Part model, mm, in its own coordinate system. Give positions to 0.01 mm unless a question says otherwise; leave off trailing zeros. Order: outer loops, then holes, each group sorted by start corner. A loop starts at its lowest first (then second) coordinate and runs counter-clockwise, first axis right, second up.
1. Slice it at C-C on x = 50. List the corners of the cut face in (y, z), and give its area (3 significant figures).
2. Slice it at B-B on y = -62. List the corners of the cut face in (x, z).
3. Probe line 1 (Y direction, x = 0, z = 8.5); line 2 (Z direction, x = 46.5, y = 59); line 3 (X direction, y = 2, z = 3.5). List the from-to ranges inside material, lowest first.
4. Drop flat-ended pins along their axis: pin 1 Ø3 at (x, y) = (-45, -10) entering from +Z; pin 2 Ø3.5 at (x, z) = (-0.5, 4) entering from +Y. Give the stop position or say it passes through.
5. Slice it at A-A on z = 4.75. List the corners of the cut face in (x, y), and give its area (3 significant figures).
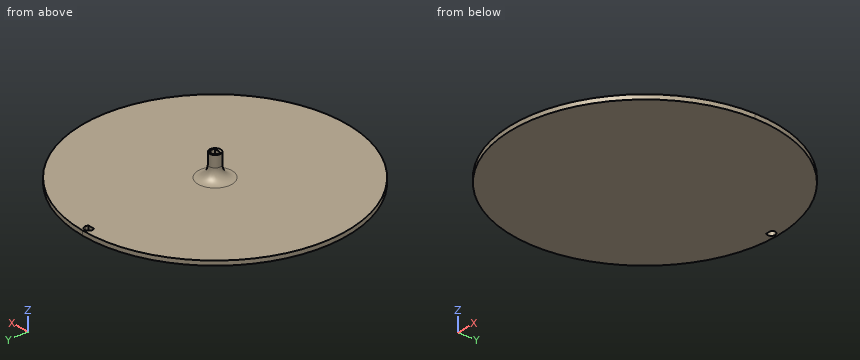
from build123d import *

# Parameters (mm, degrees)
F0_R     = 3.7
F1_DEPTH = 15
F3_DEPTH = 3


with BuildPart() as f1:
    # F0 (on Top) → F1 (new body)
    with BuildSketch(Plane.XY):
        Circle(F0_R)
        with BuildLine():
            ThreePointArc((-2.0976176963, -1.7), (-0.9017849577, 2.5449526302), (2.7, 0))
            ThreePointArc((2.7, 0), (2.5449526302, -0.9017849577), (2.0976176963, -1.7))
            ThreePointArc((2.0976176963, -1.7), (0, -2.7), (-2.0976176963, -1.7))
        make_face(mode=Mode.SUBTRACT)
        with BuildLine():
            Line((0, -1.7), (-2.0976176963, -1.7))
            ThreePointArc((-2.0976176963, -1.7), (0, -2.7), (2.0976176963, -1.7))
            Line((2.0976176963, -1.7), (0, -1.7))
        make_face()
    extrude(amount=F1_DEPTH)

    # F2 (on Top) → F3 (join)
    with BuildSketch(Plane.XY):
        with BuildLine():
            ThreePointArc((0, 87.5), (-61.8718433538, -61.8718433538), (87.5, 0))
            ThreePointArc((87.5, 0), (61.8718433538, 61.8718433538), (0, 87.5))
        make_face()
        with BuildLine():
            ThreePointArc((-2.0976176963, 81.8), (-2.4372115214, 84.6618950039), (0, 86.2))
            ThreePointArc((0, 86.2), (1.9091883092, 85.4091883092), (2.7, 83.5))
            ThreePointArc((2.7, 83.5), (2.5449526302, 82.5982150423), (2.0976176963, 81.8))
            ThreePointArc((2.0976176963, 81.8), (1.1618950039, 81.0627884786), (0, 80.8))
            ThreePointArc((0, 80.8), (-1.1618950039, 81.0627884786), (-2.0976176963, 81.8))
        make_face(mode=Mode.SUBTRACT)
        with BuildLine():
            Line((0, 81.8), (-2.0976176963, 81.8))
            ThreePointArc((-2.0976176963, 81.8), (-1.1618950039, 81.0627884786), (0, 80.8))
            Line((0, 80.8), (0, 81.8))
        make_face()
        with BuildLine():
            Line((2.0976176963, 81.8), (0, 81.8))
            Line((0, 81.8), (0, 80.8))
            ThreePointArc((0, 80.8), (1.1618950039, 81.0627884786), (2.0976176963, 81.8))
        make_face()
    extrude(amount=-F3_DEPTH)

    # F4 (on Right) → F5 (revolve)
    with BuildSketch(Plane.YZ):
        with BuildLine():
            Line((3.7, 7.5), (3.7, 0))
            Line((3.7, 0), (11.2, 0))
            ThreePointArc((11.2, 0), (5.8966991411, 2.1966991411), (3.7, 7.5))
        make_face()
    revolve(axis=Axis((0, 0, 3.75), (0, 0, 1)))


solid = f1.part
Data:
1. outline: (-71.81, -3) - (71.81, -3) - (71.81, 0) - (-71.81, 0) - close
1. area: 431 mm2
2. outline: (-61.74, -3) - (61.74, -3) - (61.74, 0) - (-61.74, 0) - close
3. line 1: y = -3.7 to -1.7, 2.7 to 3.7
3. line 2: z = -3 to 0
3. line 3: x = -4.42 to -1.81, 1.81 to 4.42
4. pin 1: stops at z = 0
4. pin 2: stops at y = 5.83
5. outline: circle Ø8.44 at (0, 0); hole (-2.1, -1.7) - (2.1, -1.7) arc R2.7 ccw (long way) to start
5. area: 36.0 mm2
